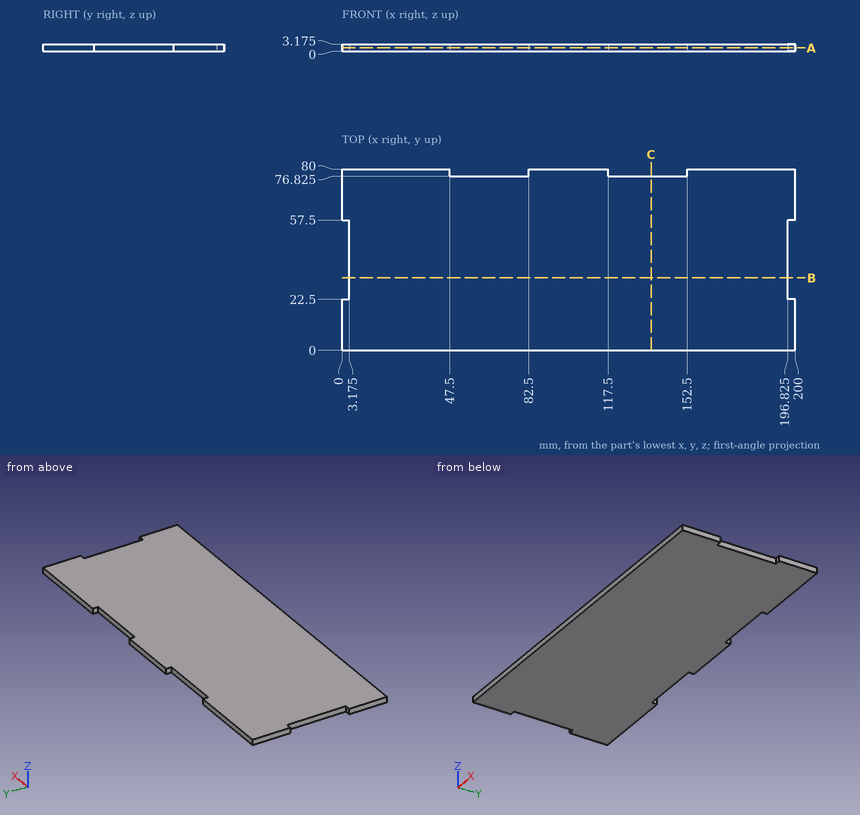
Check sheet for the drawn part. Datum: minimum x, y, z corner. Units: mm. Give positions to 0.01 mm unless a question says otherwise; leave off trailing zeros. Loops run counter-clockwise (first coordinate to the right, second up) from the corner with the lowest first, then second, coordinate; pieces in that order, holes last.
1) Depth check by flat-ended pin: pin 1 Ø1.6 at (x, z) = (59.5, 2) entering from +Y (3 decimals). Enter the tip coordinate at first touch or a pass-through.
2) Sectioned sample at B-B, the plane y = 32. Enter the section's corners in (x, z) (3 decimals), then the cut area to 3 significant figures.
3) Thickness scan on line 1 along X through (y, z) = (49, 2.7) (3 decimals); line 2 along Y through (x, z) = (53, 2.65) (3 decimals). Record the ranges inside material, lowest first.
4) Sectioned sample at C-C, the plane x = 136.5. Enter the section's corners in (y, z) (3 decimals), then the cut area to 3 significant figures.
5) Sectioned sample at A-A, the plane z = 1.45. Enter the section's corners in (x, y) (3 decimals).
Answers:
1. pin 1: stops at y = 76.825
2. outline: (3.175, 0) - (196.825, 0) - (196.825, 3.175) - (3.175, 3.175) - close
2. area: 615 mm2
3. line 1: x = 3.175 to 196.825
3. line 2: y = 0 to 76.825
4. outline: (0, 0) - (76.825, 0) - (76.825, 3.175) - (0, 3.175) - close
4. area: 244 mm2
5. outline: (0, 0) - (200, 0) - (200, 22.5) - (196.825, 22.5) - (196.825, 57.5) - (200, 57.5) - (200, 80) - (152.5, 80) - (152.5, 76.825) - (117.5, 76.825) - (117.5, 80) - (82.5, 80) - (82.5, 76.825) - (47.5, 76.825) - (47.5, 80) - (0, 80) - (0, 57.5) - (3.175, 57.5) - (3.175, 22.5) - (0, 22.5) - close
